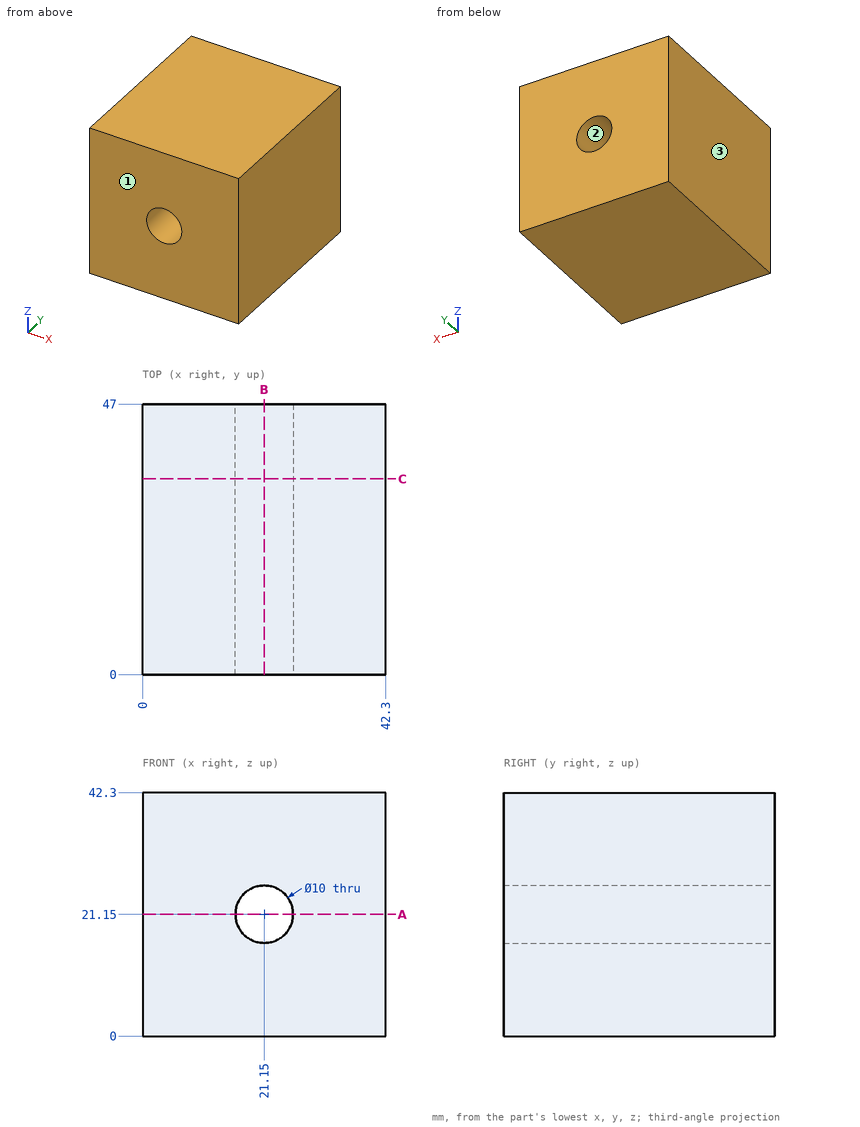
Geometry: see drawing. Coordinates: mm, zero at the bounding-box minimum. Round coordinates to 2 decimals unless told otherwise and drop trailing zeros. Write each loop counter-clockwise with the first axis right and the second up, starting at its lowest first coordinate (ties: lowest second). Pieces come first, ordered by that corner, then holes.
1) Cut plane B-B (x = 21.15). Return the cut outline in (y, z).
2) Cut plane A-A (z = 21.15). Return the cut outline in (x, y), then the cut area to 3 significant figures.
3) Cut plane C-C (y = 34). Return the cut outline in (x, z), then the cut area to 3 significant figures.
4) Ray query, L1, parallel to Z at x = 21.15, y = 29; L2, parallel to X at y = 28, z = 24. Return the intervals inside material, ascending.
5) Contact query for a flat-ended pin moving along its axis: P1, Ø12, axis at x = 6, y = 39.5, coming from the -Z side. Output: stop coordinate, or through.
6) Draft query along X for the marked faces 1, 2 and 3. Return one class per face: pulls with the +X half, pulls with the -X half, needs draft (parallel to the pull), parting line crosses it, or undercut.
Geometry says:
1. outline: (0, 0) - (47, 0) - (47, 16.15) - (0, 16.15) - close; (0, 26.15) - (47, 26.15) - (47, 42.3) - (0, 42.3) - close
2. outline: (0, 0) - (16.15, 0) - (16.15, 47) - (0, 47) - close; (26.15, 0) - (42.3, 0) - (42.3, 47) - (26.15, 47) - close
2. area: 1,520 mm2
3. outline: (0, 0) - (42.3, 0) - (42.3, 42.3) - (0, 42.3) - close; hole circle Ø10 at (21.15, 21.15)
3. area: 1,710 mm2
4. L1: z = 0 to 16.15, 26.15 to 42.3
4. L2: x = 0 to 17.04, 25.26 to 42.3
5. P1: stops at z = 0
6. face 1: needs draft
6. face 2: undercut
6. face 3: pulls with the -X half
